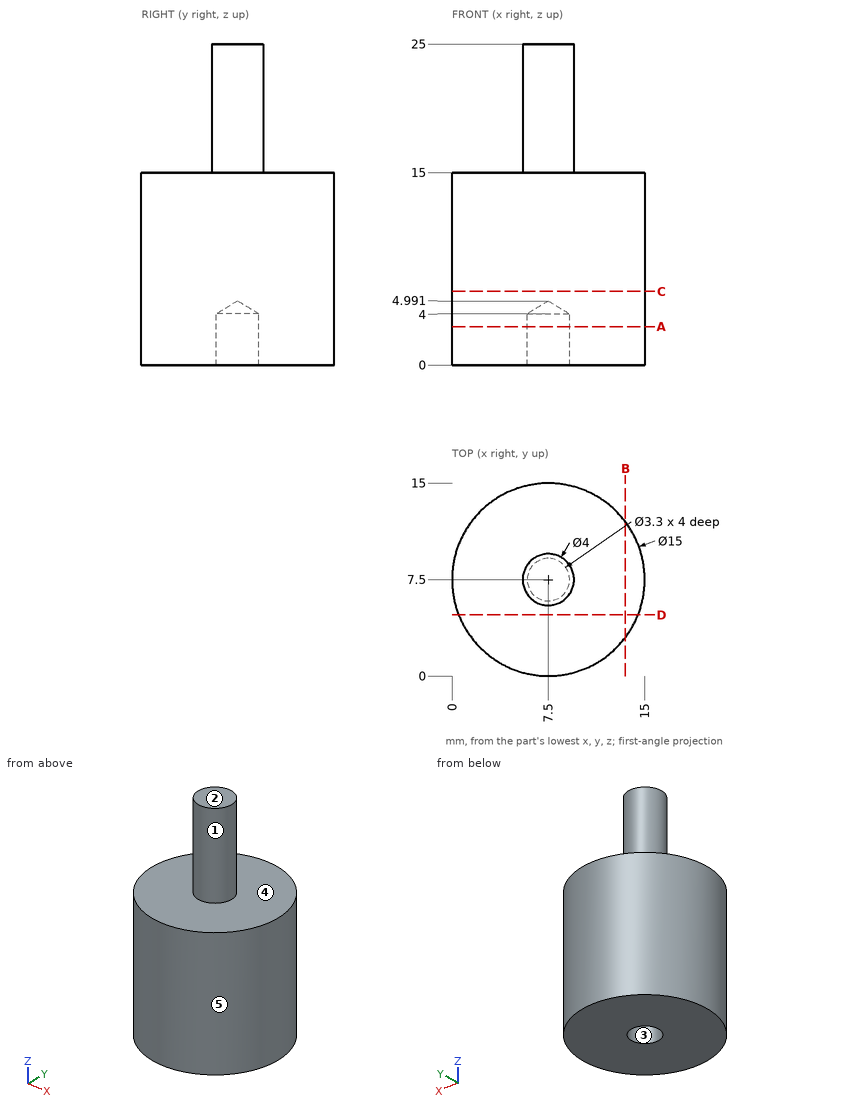
Part print with two shaded views. Sizes in mm from the minimum x, y, z corner. A direction names the side the tool comes from. Coordinates: 2 decimals unless noted, no trailing zeros. Write each loop counter-clockwise with the first axis right and the second up, starting at its lowest first coordinate (ties: lowest second). Pieces come first, ordered by that corner, then holes.
(1) Drill centre lines: line 1 (Y direction, x = 7.5, z = 2.35); line 2 (Z direction, x = 11.75, y = 11.5); line 3 (X direction, y = 7.25, z = 2.75) (1 decimal). Where is each one in solid material? Low to high.
(2) Cut at D-D on y = 4.75. List the corners of the cut face in (x, z).
(3) Mould opens along Y. For the marked faces 3, 4 and 5 say: pulls with the +Y half, pulls with the -Y half, needs draft (parallel to the pull), parting line crosses it, or undercut.
(4) Cut at A-A on z = 3. List the corners of the cut face in (x, y), and give its area (3 significant figures).
(5) Pin check, flat tips, straight feed: pin 1 Ø1.5 at (x, z) = (9.5, 6) entering from -Y (1 decimal); pin 2 Ø1 at (y, z) = (8.5, 7.5) entering from +X; pin 3 Ø6 at (x, z) = (4, 4) entering from +Y. Stop position of each tip, or through.
(6) 3-axis set-ups, long thin cutter, end or side, ignore diameter. For the marked faces 1 and 2: which of +Z, -Z, +X, -X, +Y, -Y reach the whole face in a straight line?
(7) Cut at C-C on z = 5.75. List the corners of the cut face in (x, y), and give its area (3 significant figures).
(8) Cut at B-B on x = 13.5. List the corners of the cut face in (y, z).
Working result:
1. line 1: y = 0 to 5.85, 9.15 to 15
1. line 2: z = 0 to 15
1. line 3: x = 0 to 5.9, 9.1 to 15
2. outline: (0.52, 0) - (14.48, 0) - (14.48, 15) - (0.52, 15) - close
3. face 3: undercut
3. face 4: needs draft
3. face 5: parting line crosses it
4. outline: circle Ø15 at (7.5, 7.5); hole circle Ø3.3 at (7.5, 7.5)
4. area: 168 mm2
5. pin 1: stops at y = 0.1
5. pin 2: stops at x = 14.98
5. pin 3: stops at y = 14.98
6. face 1: +Z
6. face 2: +Z, +X, -X, +Y, -Y
7. outline: circle Ø15 at (7.5, 7.5)
7. area: 177 mm2
8. outline: (3, 0) - (12, 0) - (12, 15) - (3, 15) - close
